Can you work these out from the model? Positions are in its coordinate system, mm. Round coordinates to 2 decimals unless told otherwise and drop trailing zeros. Order: outer loops, then holes, each group sorted by start corner. A loop starts at its lowest first (then second) coordinate and runs counter-clockwise, first axis right, second up. Notation, with made-up numbers: (-24, -38.75) -> (21, -38.75) arc R25 ccw to (21, -0.75) -> close; hole circle Ø1 at (-17.5, 56.25). An arc over 180 degrees is marked (long way). One line per item, written item: value.
```python
from build123d import *

# Parameters (mm, degrees)
SKETCH_W     = 900
SKETCH_H     = 1200
PAD_DEPTH    = 50
SKETCH001_W  = 75
SKETCH001_H  = 75
PAD001_DEPTH = 750
SKETCH002_W  = 75
SKETCH002_H  = 75
PAD002_DEPTH = 750
SKETCH003_W  = 75
SKETCH003_H  = 75
PAD003_DEPTH = 750
SKETCH004_W  = 75
SKETCH004_H  = 75
PAD004_DEPTH = 750


with BuildPart() as part:
    # Sketch → Pad (new body)
    with BuildSketch(Plane.XZ):
        with Locations((450, 600)):
            Rectangle(SKETCH_W, SKETCH_H)
    extrude(amount=PAD_DEPTH)

    # Sketch001 → Pad001 (join)
    with BuildSketch(Plane.XZ):
        with Locations((37.5, 37.5)):
            Rectangle(SKETCH001_W, SKETCH001_H)
    extrude(amount=PAD001_DEPTH)

    # Sketch002 → Pad002 (join)
    with BuildSketch(Plane.XZ):
        with Locations((44.296024, 1151.794312)):
            Rectangle(SKETCH002_W, SKETCH002_H)
    extrude(amount=PAD002_DEPTH)

    # Sketch003 → Pad003 (join)
    with BuildSketch(Plane.XZ):
        with Locations((854.802246, 1146.189819)):
            Rectangle(SKETCH003_W, SKETCH003_H)
    extrude(amount=PAD003_DEPTH)

    # Sketch004 → Pad004 (join)
    with BuildSketch(Plane.XZ):
        with Locations((854.802002, 42.086505)):
            Rectangle(SKETCH004_W, SKETCH004_H)
    extrude(amount=PAD004_DEPTH)


solid = part.part
```
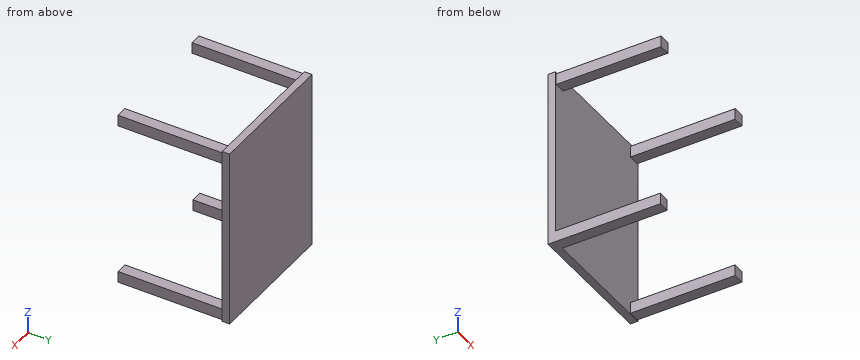
Q1. Will these pins go through, and if not, where does the flat tip stop? pin 1 Ø6 at (x, z) = (309, 617.5) entering from +Y; pin 2 Ø2 at (x, z) = (229, 162) entering from -Y; pin 3 Ø22.5 at (y, z) = (-482.5, 34.5) entering from +X.
Answers below:
pin 1: y = 0
pin 2: y = -50
pin 3: x = 892.3
Q2. I want a section at A-A on y = -638.5. List the corners of the cut face in (x, z) for me, plus the area to 3 significant figures.
Answers below:
outline: (0, 0) -> (75, 0) -> (75, 75) -> (0, 75) -> close; (6.8, 1114.29) -> (81.8, 1114.29) -> (81.8, 1189.29) -> (6.8, 1189.29) -> close; (817.3, 4.59) -> (892.3, 4.59) -> (892.3, 79.59) -> (817.3, 79.59) -> close; (817.3, 1108.69) -> (892.3, 1108.69) -> (892.3, 1183.69) -> (817.3, 1183.69) -> close
area: 22,500 mm^2
Q3. I want a section at C-C on z = 108. List the corners of the cut face in (x, y) for me, plus the area to 3 significant figures.
Answers below:
outline: (0, -50) -> (900, -50) -> (900, 0) -> (0, 0) -> close
area: 45,000 mm^2
Q4. Please list where these lines run through material, in increasing order: line 1 along Z through (x, y) = (823, -76.5); line 2 along Y through (x, z) = (349, 1147); line 3 along X through (y, z) = (-84.5, 62).
Answers below:
line 1: 4.59 to 79.59, 1108.69 to 1183.69
line 2: -50 to 0
line 3: 0 to 75, 817.3 to 892.3
Q5. I want a section at B-B on x = 796. List the corners of the cut face in (y, z) for me.
Answers below:
outline: (-50, 0) -> (0, 0) -> (0, 1200) -> (-50, 1200) -> close
